The listing builds one solid part. Answer for the finished solid, in the listing's coordinates (mm). A direction names the side the tool comes from. Coordinates: 2 decimals unless noted, no trailing zeros. Write each loop counter-clockwise with the first axis right and the second up, starting at its lowest first coordinate (ties: lowest second). Pieces come first, ordered by that corner, then holes.
(1) Given P1, Ø6, axis at x = -5, y = -8, coming from the +Z side; P2, Ø13.5, axis at y = -3.5, z = -51, coming from the -X side; P3, Ø10, axis at x = 2.5, y = -18, coming from the -Z side; P4, Ø3, axis at x = -16.5, z = -17, coming from the +Y side, each flat-ended and moving along its own axis, determine where each tip first touches the part or whether it passes through.
(2) The part is cut by section C-C on z = 8.5. Determine the outline of the cut face in (x, y).
(3) The part is cut by section A-A on z = -45. Determine the outline of the cut face in (x, y), plus the area to 3 significant figures.
(4) The part is cut by section D-D on x = -26.5. Determine the outline of the cut face in (y, z), plus the area to 3 significant figures.
(5) Straight lines are drawn through the part: line 1 (X direction, y = -3, z = -49); line 2 (Z direction, x = -15.5, y = -21.75); line 3 (Y direction, x = -11.5, z = -25.5). For each, find the intervals that lie inside material, in ascending order.
(6) The part is cut by section B-B on y = -4.25. Determine the outline of the cut face in (x, z), plus the area to 3 significant figures.
(7) Which of the six approach directions +Z, -Z, +X, -X, +Y, -Y give full straight-line access (tool end or side, diameter ignored) to faces 4 (the flat face through (-9, -25.4, 30)), 5 (the flat face through (-47.357, -10, -6)), 6 (the flat face through (-14.884, -6, -50)), 7 (the flat face through (-9, -12.7, -33)), 8 (the flat face through (30.956, -10, -7))?
(8) For a pull along Z with two mould halves and no side action, classify faces 1 (the cylindrical face through (-15.592, -12.522, 10.918)), 2 (the flat face through (-18, 0, 8)), 3 (the flat face through (14, -6, -55.868)) as +Z half, -Z half, draft (parallel to the pull), parting line (faces both ways), or undercut.
from build123d import *

# Parameters (mm, degrees)
F1_DEPTH = 12.7
F3_DEPTH = 12.7
F5_D     = 16.002


with BuildPart() as f1:
    # F0 (on Front) → F1 (new body)
    with BuildSketch(Plane.XZ):
        with BuildLine():
            Line((-47.357348, 25.225591), (-47.357348, -19.035261))
            Line((-47.357348, -19.035261), (-47.357348, -55.867718))
            Line((-47.357348, -55.867718), (-14.88383, -55.867718))
            Line((-14.88383, -55.867718), (-14.88383, -43.249417))
            ThreePointArc((-14.88383, -43.249417), (-14.884202, -43.178936), (-14.88383, -43.108455))
            ThreePointArc((-14.88383, -43.108455), (-8.260409, -36.49587), (-1.520228, -42.989401))
            ThreePointArc((-1.520228, -42.989401), (-1.51754, -43.178936), (-1.520228, -43.368471))
            Line((-1.520228, -43.368471), (-1.520228, -55.867718))
            Line((-1.520228, -55.867718), (30.955606, -55.867718))
            Line((30.955606, -55.867718), (30.955606, 25.225591))
            ThreePointArc((30.955606, 25.225591), (-8.200871, 70.891809), (-47.357348, 25.225591))
        make_face()
    extrude(amount=F1_DEPTH)

    # F2 (on face) → F3 (join)
    with BuildSketch(Plane.XZ.offset(12.7)):
        with BuildLine():
            Line((-47.357348, 25.225591), (-47.357348, -11.417718))
            Line((-47.357348, -11.417718), (30.955606, -11.417718))
            Line((30.955606, -11.417718), (30.955606, 25.225591))
            ThreePointArc((30.955606, 25.225591), (-8.200871, 70.891809), (-47.357348, 25.225591))
        make_face()
    extrude(amount=F3_DEPTH)

    # F5 (through all)
    with Locations(Plane.XZ.offset(25.4)):
        with Locations((-8.200871, 13.982282)):
            Hole(F5_D / 2)


solid = f1.part
Model answer:
1. P1: stops at z = 70.89
1. P2: stops at x = -47.36
1. P3: stops at z = -11.42
1. P4: stops at y = 0
2. outline: (-47.36, -25.4) - (-14.03, -25.4) - (-14.03, 0) - (-47.36, 0) - close; (-2.37, -25.4) - (30.96, -25.4) - (30.96, 0) - (-2.37, 0) - close
3. outline: (-47.36, -12.7) - (-14.88, -12.7) - (-14.88, 0) - (-47.36, 0) - close; (-1.52, -12.7) - (30.96, -12.7) - (30.96, 0) - (-1.52, 0) - close
3. area: 825 mm2
4. outline: (-25.4, -11.42) - (-12.7, -11.42) - (-12.7, -55.87) - (0, -55.87) - (0, 66.41) - (-25.4, 66.41) - close
4. area: 2,540 mm2
5. line 1: x = -47.36 to -14.88, -1.52 to 30.96
5. line 2: z = -11.42 to 10.71, 17.26 to 70.21
5. line 3: y = -12.7 to 0
6. outline: (-47.36, -55.87) - (-14.88, -55.87) - (-14.88, -43.25) arc R6.68 cw to (-14.88, -43.11) arc R6.68 cw to (-1.52, -42.99) arc R6.68 cw to (-1.52, -43.37) - (-1.52, -55.87) - (30.96, -55.87) - (30.96, 25.23) arc R39.62 ccw (long way) to (-47.36, 25.23) - close; hole circle Ø16 at (-8.2, 13.98)
6. area: 8,850 mm2
7. face 4: +Z, -Z, +X, -X, -Y
7. face 5: -Z, -X, +Y, -Y
7. face 6: -Z, +Y, -Y
7. face 7: -Z, +X, -X, -Y
7. face 8: -Z, +X, +Y, -Y
8. face 1: undercut
8. face 2: draft
8. face 3: -Z half
